```python
from build123d import *

# Parameters (mm, degrees)
F1_DEPTH = 12.5
F6_R     = 2.5
F7_DEPTH = 3


with BuildPart() as f1:
    # F0 (on Top) → F1 (new body, symmetric)
    with BuildSketch(Plane.XY):
        with BuildLine():
            Line((0, 0), (31.985281, 0))
            Line((31.985281, 0), (31.985281, 4.529437))
            ThreePointArc((31.985281, 4.529437), (32.746486, 8.356272), (34.914214, 11.600505))
            Line((34.914214, 11.600505), (75.942641, 52.628932))
            Line((75.942641, 52.628932), (75.942641, 57.582843))
            Line((75.942641, 57.582843), (72.267767, 61.257716))
            ThreePointArc((72.267767, 61.257716), (71.914214, 61.404163), (71.56066, 61.257716))
            Line((71.56066, 61.257716), (69.236437, 58.933493))
            ThreePointArc((69.236437, 58.933493), (69.08999, 58.57994), (69.236437, 58.226386))
            Line((69.236437, 58.226386), (69.377858, 58.084965))
            ThreePointArc((69.377858, 58.084965), (69.731411, 57.938518), (70.084965, 58.084965))
            Line((70.084965, 58.084965), (70.5, 58.5))
            Line((70.5, 58.5), (71.914214, 59.914214))
            Line((71.914214, 59.914214), (74.742641, 57.085786))
            Line((74.742641, 57.085786), (73.328427, 55.671573))
            Line((73.328427, 55.671573), (26.328427, 8.671573))
            Line((26.328427, 8.671573), (23.5, 11.5))
            Line((23.5, 11.5), (23.707107, 11.707107))
            ThreePointArc((23.707107, 11.707107), (23.815493, 12.252002), (23.353553, 12.56066))
            Line((23.353553, 12.56066), (18.370521, 12.56066))
            ThreePointArc((18.370521, 12.56066), (0, 6), (-18.370521, 12.56066))
            Line((-18.370521, 12.56066), (-23.353553, 12.56066))
            ThreePointArc((-23.353553, 12.56066), (-23.815493, 12.252002), (-23.707107, 11.707107))
            Line((-23.707107, 11.707107), (-23.5, 11.5))
            Line((-23.5, 11.5), (-26.328427, 8.671573))
            Line((-26.328427, 8.671573), (-73.328427, 55.671573))
            Line((-73.328427, 55.671573), (-74.742641, 57.085786))
            Line((-74.742641, 57.085786), (-71.914214, 59.914214))
            Line((-71.914214, 59.914214), (-70.5, 58.5))
            Line((-70.5, 58.5), (-70.084965, 58.084965))
            ThreePointArc((-70.084965, 58.084965), (-69.731411, 57.938518), (-69.377858, 58.084965))
            Line((-69.377858, 58.084965), (-69.236437, 58.226386))
            ThreePointArc((-69.236437, 58.226386), (-69.08999, 58.57994), (-69.236437, 58.933493))
            Line((-69.236437, 58.933493), (-71.56066, 61.257716))
            ThreePointArc((-71.56066, 61.257716), (-71.914214, 61.404163), (-72.267767, 61.257716))
            Line((-72.267767, 61.257716), (-75.942641, 57.582843))
            Line((-75.942641, 57.582843), (-75.942641, 52.628932))
            Line((-75.942641, 52.628932), (-34.914214, 11.600505))
            ThreePointArc((-34.914214, 11.600505), (-32.746486, 8.356272), (-31.985281, 4.529437))
            Line((-31.985281, 4.529437), (-31.985281, 0))
            Line((-31.985281, 0), (0, 0))
        make_face()
    extrude(amount=F1_DEPTH, both=True)


with BuildPart() as f3:
    # F2 (on Top) → F3 (revolve)
    with BuildSketch(Plane.XY):
        Polygon((-18, 19.219435), (-18, -4.799377), (-16.75, -4.799377), (-16.75, 7), (-14.75, 7), (-14.75, 19.219435), align=None)
    revolve(axis=Axis((-18, 7.210029, 0), (0, -1, 0)))


with BuildPart() as f4_1:
    # F4: instance of F3
    add(f3.part.mirror(Plane.YZ))


with BuildPart() as f1_1:
    add(f1.part)

    # F5: cut F3, F4_1
    add(f3.part, mode=Mode.SUBTRACT)
    add(f4_1.part, mode=Mode.SUBTRACT)

    # F6 (on face) → F7 (join)
    with BuildSketch(Plane(origin=(0, 0, -12.5), x_dir=(1, 0, 0), z_dir=(0, 0, -1))):
        Polygon((46.985281, 15), (0, 15), (0, 0), (23.313708, 0), (75.942641, -52.628932), align=None)
        with Locations((26.328427, 7.5)):
            Circle(F6_R, mode=Mode.SUBTRACT)
        Polygon((0, 0), (0, 15), (-46.985281, 15), (-75.942641, -52.628932), (-23.313708, 0), align=None)
        with Locations((-26.328427, 7.5)):
            Circle(F6_R, mode=Mode.SUBTRACT)
    extrude(amount=-F7_DEPTH)


solid = f1_1.part
```
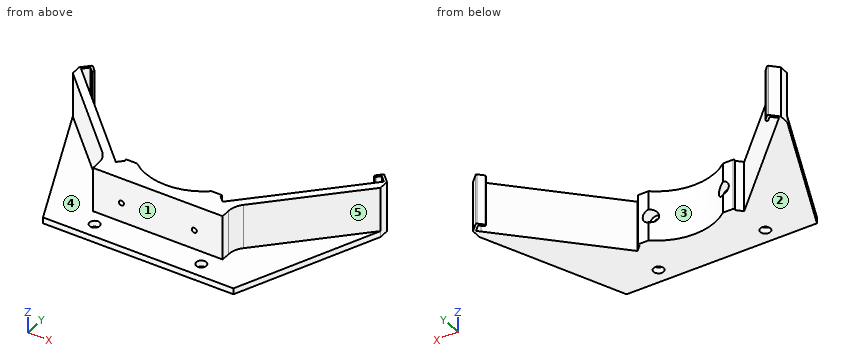
Here's how the part is built. I have some questions about the finished solid (model axes, mm). Face numbers are marked on the shaded views. A direction names the side the tool comes from. Give positions to 0.01 mm unless a question says otherwise; leave off trailing zeros. Write each loop counter-clockwise with the first axis right and the second up, starting at its lowest first coordinate (ties: lowest second). Pieces come first, ordered by that corner, then holes. Notation, with made-up numbers: (19.25, -27) -> (70.25, -27) arc R25 cw to (70.25, -2) -> close; hole circle Ø5 at (-1.75, -12.5). An arc over 180 degrees is marked (long way). Write each question's results on one line, items separated by ' | '.
Item 1: We'd pull the mould along X, two halves only. Please class the marked faces 3, 4 and 5: pulls with the +X half, pulls with the -X half, needs draft (parallel to the pull), parting line crosses it, or undercut.
Output:
face 3: undercut | face 4: needs draft | face 5: pulls with the +X half
Item 2: If I drill on L1, parallel to Z at x = 18, y = 4; L2, parallel to X at y = -7.5, z = -11.9; L3, parallel to Y at x = -22, z = -8.75, over which ranges is the centre line in solid material (lowest first)?
Output:
L1: z = -12.5 to -1.25, 1.25 to 12.5 | L2: x = -50.2 to -28.83, -23.83 to 23.83, 28.83 to 50.2 | L3: y = 0 to 12.56
Item 3: Suppose I cut it at D-D on x = -49.5. Write out the boundary of the cut face in (y, z), plus the area to 3 significant figures.
Output:
outline: (-9.13, -12.5) -> (31.84, -12.5) -> (31.84, 12.5) -> (26.19, 12.5) -> (26.19, -9.5) -> (-9.13, -9.5) -> close | area: 247 mm^2
Item 4: For pin 1 Ø4 at (x, y) = (-26.33, -7.5) entering from -Z; pin 2 Ø6 at (x, y) = (26.33, -7.5) entering from +Z; pin 3 Ø2 at (y, z) = (39, 2) entering from -X; pin 4 Ø6 at (y, z) = (2.5, -6) entering from +X, each with a flat end and sliding along its axis, tell me the tip position at first contact or that it passes through.
Output:
pin 1: passes through | pin 2: stops at z = -9.5 | pin 3: stops at x = -63.31 | pin 4: stops at x = 32.03
Item 5: On a 3-axis mill with a long thin cutter (end or side, diameter ignored), from which of +Z, -Z, +X, -X, +Y, -Y can I reach the whole of each face in a straight line? I mean the marked faces 1 and 2. Say none if no direction works.
Output:
face 1: +Z, +X, -X, -Y | face 2: -Z, +X, -X, +Y, -Y
Item 6: Suppose I cut it at A-A on y = -7.5. Write out the boundary of the cut face in (x, z).
Output:
outline: (-50.2, -12.5) -> (-28.83, -12.5) -> (-28.83, -9.5) -> (-50.2, -9.5) -> close; (-23.83, -12.5) -> (23.83, -12.5) -> (23.83, -9.5) -> (-23.83, -9.5) -> close; (28.83, -12.5) -> (50.2, -12.5) -> (50.2, -9.5) -> (28.83, -9.5) -> close
Item 7: Suppose I cut it at C-C on x = 59. Write out the boundary of the cut face in (y, z).
Output:
outline: (13.06, -12.5) -> (41.34, -12.5) -> (41.34, 12.5) -> (35.69, 12.5) -> (35.69, -9.5) -> (13.06, -9.5) -> close
Item 8: Suppose I cut it at B-B on y = 1.5. Write out the boundary of the cut face in (x, z), plus the area to 3 significant figures.
Output:
outline: (-54.05, -12.5) -> (54.05, -12.5) -> (54.05, -9.5) -> (31.99, -9.5) -> (31.99, 12.5) -> (-31.99, 12.5) -> (-31.99, -9.5) -> (-54.05, -9.5) -> close; hole circle Ø2.5 at (-18, 0); hole circle Ø2.5 at (18, 0) | area: 1,720 mm^2
